Autodesk Inventor part; units mm, degrees
ref_plane "YZ Plane" through (0, 0, 0) normal (1, 0, 0) x (0, 1, 0)
ref_plane "XZ Plane" through (0, 0, 0) normal (0, 1, 0) x (-1, 0, 0)
ref_plane "XY Plane" through (0, 0, 0) normal (0, 0, 1) x (1, 0, 0)
sketch "Sketch1" plane through (0, 0, 0) normal (0, 0, 1) x (1, 0, 0)
  line L0 (0, 0) -> (200, 0)
  line L1 (200, 0) -> (200, 10)
  line L2 (200, 10) -> (0, 10)
  line L3 (0, 10) -> (0, 0)
  dimension "d0" = 200
  dimension "d1" = 10
extrude "Extrusion1" add sketch "Sketch1" along normal blind 50
sketch "Sketch2" plane through (0, 10, 0) normal (0, 1, 0) x (1, 0, 0)
  line L0 (200, 0) -> (200, -50)
  line L1 (200, -23) -> (-0.0003, -23)
  line L2 (200, 0) -> (0, 0)
  line L3 (100, 0) -> (100, -50)
  line L4 (200, -50) -> (0, -50)
  circle A0 centre (81.9998, -23) radius 2.5
  circle A1 centre (117.9998, -23) radius 2.5
  point P0 (99.9998, -23)
  dimension "d4" = 23
  dimension "d5" = 5
  dimension "d6" = 5
  dimension "d7" = 18
  dimension "d8" = 36
sketch "Sketch3" plane through (0, 0, 0) normal (0, 0, -1) x (-1, 0, 0)
  line L0 (0, 0) -> (-200, 0)
  line L1 (-200, 10) -> (0, 10)
  line L2 (0, 0) -> (-200, 0)
  line L3 (-200, 0) -> (-200, 10)
  line L4 (-200, 10) -> (0, 10)
  line L5 (0, 10) -> (0, 0)
extrude "Extrusion3" add sketch "Sketch3" along normal blind 10
sketch "Sketch4" plane through (0, 10, 50) normal (0, 1, 0) x (1, 0, 0)
  line L0 (0, 0) -> (200, 0)
  line L1 (100, 0) -> (100, 60)
  line L2 (0, 60) -> (200, 60)
  circle A0 centre (100, 27) radius 5
  point P0 (0, 50)
  dimension "d17" = 10
  dimension "d39" = 33
extrude "Extrusion4" cut sketch "Sketch4" against normal blind 10
sketch "Sketch5" plane through (0, 0, 50) normal (0, -1, 0) x (1, 0, 0)
  line L0 (140, -40) -> (140, -50)
  line L1 (140, -50) -> (60, -50)
  line L2 (60, -50) -> (60, -40)
  line L3 (0, -40) -> (60, -40)
  line L4 (0, -60) -> (0, -40)
  line L5 (0, -60) -> (200, -60)
  line L6 (200, -60) -> (200, -40)
  line L7 (140, -40) -> (200, -40)
  circle A0 centre (30, -50) radius 2.4585
  circle A1 centre (170, -50) radius 2.4585
  point P0 (0, -50)
  point P1 (170, -50)
  point P2 (30, -50)
  point P3 (200, -50)
  point P4 (170, -40)
  point P5 (30, -40)
hole "Hole1" at (170, 0, 0) at (30, 0, 0) direction (0, 1, 0) diameter 6.5 end through all counterbore diameter 11 counterbore depth 5
hole "Hole2" at (81.9998, 10, 23) at (117.9998, 10, 23) direction (0, -1, 0) diameter 4.134 end through all
sketch "Sketch6" plane through (0, 10, 50) normal (0, 1, 0) x (1, 0, 0)
  line L0 (200, 0) -> (0, 0)
  line L1 (0, 0) -> (200, 0)
  line L2 (200, 0) -> (200, 10)
  line L3 (200, 10) -> (0, 10)
  line L4 (0, 10) -> (0, 0)
  point P0 (0, 50)
  dimension "d35" = 10
extrude "Extrusion5" cut sketch "Sketch6" against normal through all
sketch "Sketch7" plane through (0, 10, -10) normal (0, 1, 0) x (1, 0, 0)
  point P0 (0, -10)
fillet "Fillet3" radius 5 2 edges at (0, 5, 40) (200, 5, 40)
properties part number "Nap_duoi"
Input: part model. Units: mm. Frame: model coordinates. A direction names the side the tool comes from. Round coordinates to 2 decimals unless told otherwise and drop trailing zeros. Loops run counter-clockwise (first coordinate to the right, second up) from the corner with the lowest first, then second, coordinate; pieces in that order, holes last. Notation, with made-up numbers: (17, -0.5) -> (36, -0.5) arc R22 ccw to (36, 17.5) -> close; hole circle Ø9 at (-15.5, 44). An arc over 180 degrees is marked (long way). One line per item, written item: value.
(1) Material intervals for line 1 (X direction, y = 2.55, z = 0); line 2 (X direction, y = 3, z = 23); line 3 (X direction, y = 8.8, z = 0), sorted ascending. Write a range as [from, to].
Geometry check:
line 1: [0, 24.5], [35.5, 164.5], [175.5, 200]
line 2: [0, 79.93], [84.07, 95], [105, 115.93], [120.07, 200]
line 3: [0, 26.75], [33.25, 166.75], [173.25, 200]
(2) Section A-A (z = 23). Return the cut outline in (x, y).
Geometry check:
outline: (0, 0) -> (79.93, 0) -> (79.93, 10) -> (0, 10) -> close; (84.07, 0) -> (95, 0) -> (95, 10) -> (84.07, 10) -> close; (105, 0) -> (115.93, 0) -> (115.93, 10) -> (105, 10) -> close; (120.07, 0) -> (200, 0) -> (200, 10) -> (120.07, 10) -> close
(3) Set-up query: faces 1 (the face through (99, 0, 15)), 2 (the face through (175.37, 2.54, 1.19)). Return all of +Z, -Z, +X, -X, +Y, -Y with unobstructed straight access to the full face (end or side cutting, diameter ignored); none if empty.
Geometry check:
face 1: +Z, -Z, +X, -X, -Y
face 2: -Y
(4) Section B-B (z = 0). Return the cut outline in (x, y), plus the area to 4 significant figures.
Geometry check:
outline: (0, 0) -> (24.5, 0) -> (24.5, 5) -> (26.75, 5) -> (26.75, 10) -> (0, 10) -> close; (33.25, 5) -> (35.5, 5) -> (35.5, 0) -> (164.5, 0) -> (164.5, 5) -> (166.75, 5) -> (166.75, 10) -> (33.25, 10) -> close; (173.25, 5) -> (175.5, 5) -> (175.5, 0) -> (200, 0) -> (200, 10) -> (173.25, 10) -> close
area: 1,825 mm2
(5) Section C-C (x = 30). Return the cut outline in (y, z).
Geometry check:
outline: (0, -10) -> (10, -10) -> (10, -3.25) -> (5, -3.25) -> (5, -5.5) -> (0, -5.5) -> close; (0, 5.5) -> (5, 5.5) -> (5, 3.25) -> (10, 3.25) -> (10, 40) -> (0, 40) -> close
(6) Section D-D (x = 99). Return the cut outline in (y, z), plus the area to 3 significant figures.
Geometry check:
outline: (0, -10) -> (10, -10) -> (10, 18.1) -> (0, 18.1) -> close; (0, 27.9) -> (10, 27.9) -> (10, 40) -> (0, 40) -> close
area: 402 mm2
(7) Mould query, pull axis X, two halves, no side actions, for faces 3 (the face through (199, 5, 38)), 4 (the face through (104.619, 5.07, 24.915)), 5 (the face through (101, 10, 15)). Classes: pulls with the +X half, pulls with the -X half, needs draft (parallel to the pull), parting line crosses it, or undercut.
Geometry check:
face 3: pulls with the +X half
face 4: undercut
face 5: needs draft
(8) Pin query (flat end, axial travel): pin 1 (3.5 mm diameter, centred on x = 30, z = 2.5, fed in from -Y); pin 2 (8 mm diameter, centred on x = 100, z = 23, fed in from -Y). Return the tip coordinate at first contact, or that it passes through.
Geometry check:
pin 1: y = 5
pin 2: through
